Can you work these out from the model? Positions are in its coordinate system, mm. Face numbers are marked on the shaded views. A direction names the side the tool comes from. Coordinates: 2 decimals unless noted, no trailing zeros. Loops run counter-clockwise (first coordinate to the right, second up) from the corner with the lowest first, then second, coordinate; pieces in that order, holes last. Notation, with made-up numbers: (60, 23.5) - (97, 23.5) arc R24 cw to (97, 54.5) - close; hole circle Ø6 at (72.25, 43.5). An arc over 180 degrees is marked (long way). Put each result on its own line as item: value. Start each with the question number.
from build123d import *

# Parameters (mm, degrees)
SKETCH1_R           = 0.75
BOSS_EXTRUDE1_DEPTH = 9.5
CUT_EXTRUDE1_DEPTH  = 8.5


with BuildPart() as part:
    # Sketch1 → Boss-Extrude1 (new, symmetric)
    with BuildSketch(Plane.XY):
        with BuildLine():
            Line((0, -1), (0, -22.957082326))
            ThreePointArc((0, -22.957082326), (-0.687794809, -23.907097019), (-1.805055837, -23.550281364))
            Line((-1.805055837, -23.550281364), (-13.805055837, -7.264567078))
            ThreePointArc((-13.805055837, -7.264567078), (-13.950014694, -6.983573231), (-14, -6.67136804))
            Line((-14, -6.67136804), (-14, -1))
            ThreePointArc((-14, -1), (-13.707106781, -0.292893219), (-13, 0))
            Line((-13, 0), (-1, 0))
            ThreePointArc((-1, 0), (-0.292893219, -0.292893219), (0, -1))
        make_face()
        with Locations((-11, -3)):
            Circle(SKETCH1_R, mode=Mode.SUBTRACT)
        with Locations((-3, -3)):
            Circle(SKETCH1_R, mode=Mode.SUBTRACT)
    extrude(amount=BOSS_EXTRUDE1_DEPTH, both=True)

    # Sketch2 → Cut-Extrude1 (cut, symmetric)
    with BuildSketch(Plane.XY):
        Polygon((-1, -28.348579048), (-1, -6.907097019), (7.926418822, -6.907097019), (7.294916487, 4.746991522), (-21.667349138, 6.871135739), (-20.03469418, -23.258769395), align=None)
    extrude(amount=CUT_EXTRUDE1_DEPTH, both=True, mode=Mode.SUBTRACT)


solid = part.part
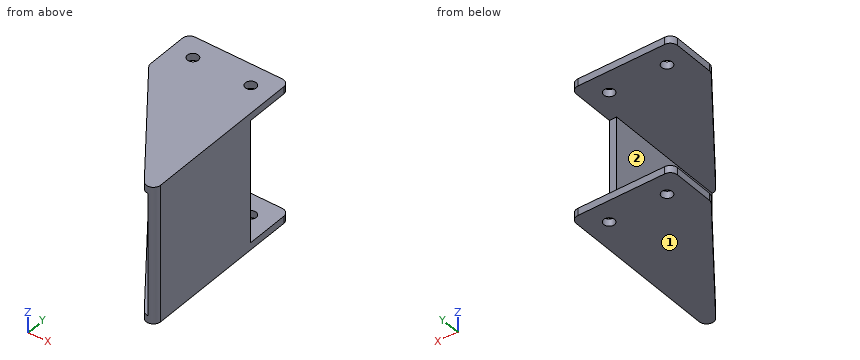
Q1. I want a section at C-C on y = -16.5. List the corners of the cut face in (x, z) for me, and give its area (3 significant figures).
Q2. Will these pins go through, and if not, where does the flat tip stop? pin 1 (8 mm diameter, centred on y = -11, z = -2.5, fed in from -X); pin 2 (0.5 mm diameter, centred on x = -0.5, z = 2.5, fed in from +Y).
Q3. On a 3-axis mill with a long thin cutter (end or side, diameter ignored), from which of +Z, -Z, +X, -X, +Y, -Y can I reach the whole of each face in a straight line? I mean the marked faces 1 and 2. Say none if no direction works.
Q4. I want a section at A-A on y = -3. List the corners of the cut face in (x, z) for me.
Q5. Please list where these lines run through material, in increasing order: line 1 along X through (y, z) = (-3, -8.95); line 2 along Z through (x, y) = (-2, -18.75); line 3 along X through (y, z) = (-9.25, -3.25). Write a range as [from, to].
Q6. I want a section at D-D on z = 4.25. List the corners of the cut face in (x, y) for me, and give its area (3 significant figures).
Q7. I want a section at B-B on x = -11. List the corners of the cut face in (y, z) for me, and give its area (3 significant figures).
Calculated:
1. outline: (-7, -9.5) - (0, -9.5) - (0, 9.5) - (-7, 9.5) - (-7, 8.5) - (-1, 8.5) - (-1, -8.5) - (-7, -8.5) - close
1. area: 31.0 mm2
2. pin 1: x = -1
2. pin 2: y = -6.91
3. face 1: -Z, +X, -X, +Y, -Y
3. face 2: -X, +Y, -Y
4. outline: (-14, -9.5) - (-11.75, -9.5) - (-11.75, -8.5) - (-14, -8.5) - close; (-14, 8.5) - (-11.75, 8.5) - (-11.75, 9.5) - (-14, 9.5) - close; (-10.25, -9.5) - (-3.75, -9.5) - (-3.75, -8.5) - (-10.25, -8.5) - close; (-10.25, 8.5) - (-3.75, 8.5) - (-3.75, 9.5) - (-10.25, 9.5) - close; (-2.25, -9.5) - (0, -9.5) - (0, -8.5) - (-2.25, -8.5) - close; (-2.25, 8.5) - (0, 8.5) - (0, 9.5) - (-2.25, 9.5) - close
5. line 1: [-14, -11.75], [-10.25, -3.75], [-2.25, 0]
5. line 2: [-9.5, -8.5], [8.5, 9.5]
5. line 3: [-1, 0]
6. outline: (-1, -23.96) arc R1 ccw to (0, -22.96) - (0, -6.91) - (-1, -6.91) - close
6. area: 16.8 mm2
7. outline: (-11.07, -9.5) - (-3.75, -9.5) - (-3.75, -8.5) - (-11.07, -8.5) - close; (-11.07, 8.5) - (-3.75, 8.5) - (-3.75, 9.5) - (-11.07, 9.5) - close; (-2.25, -9.5) - (0, -9.5) - (0, -8.5) - (-2.25, -8.5) - close; (-2.25, 8.5) - (0, 8.5) - (0, 9.5) - (-2.25, 9.5) - close
7. area: 19.1 mm2
